Design review of the part built by this model. Coordinates are the model's own, in mm. Face numbers are marked on the shaded views. Coordinates: 2 decimals unless noted, no trailing zeros. Loops run counter-clockwise (first coordinate to the right, second up) from the corner with the lowest first, then second, coordinate; pieces in that order, holes last. Notation, with made-up numbers: (24, 15) -> (56, 15) arc R28 cw to (56, 34) -> close; hole circle Ø4 at (-32.75, 84). An arc over 180 degrees is marked (long way). One line per item, written item: value. Start each with the question number.
1. Insertion check: pin 1 (1.2 mm diameter, centred on x = 2.67, z = -5.07, fed in from +Y). The pin has a flat end and moves straight along its axis. Give the tip position at first contact, or say it passes through.
2. For probe 1 along Z at (x, y) = (2.6, 0.85); probe 2 along Z at (x, y) = (2.45, 1.7); probe 3 along X at (y, z) = (2.45, -25), list the stretches that pass through material, from the lowest coordinate up.
3. Add section C-C on y = 2.55. Write out the cut boundary in (x, z).
4. Add section B-B on x = 2.6. Write out the cut boundary in (y, z).
5. Draft analysis for pull direction Z (two halves, no side actions). For the marked faces 1, 2 and 3, state which applies: pulls with the +Z half, pulls with the -Z half, needs draft (parallel to the pull), parting line crosses it, or undercut.
6. Add section A-A on z = -25. Write out the cut boundary in (x, y).
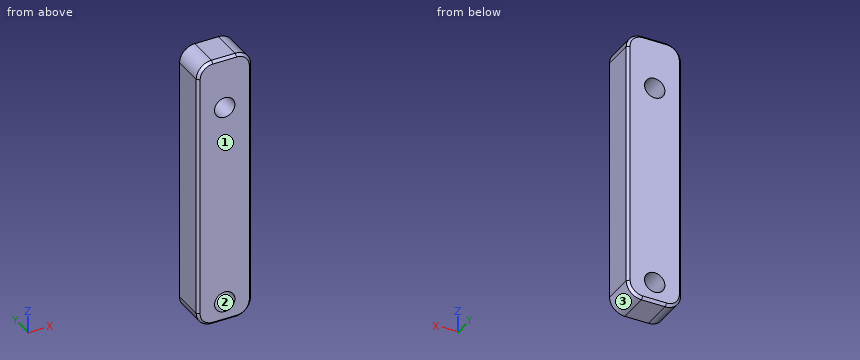
```python
from build123d import *

# Parameters (mm, degrees)
SKETCH_1_W          = 5.332575
SKETCH_1_H          = 27
EXTRUDE_1_DEPTH     = 3.5
FILLET_1_R          = 1.5
SKETCH_2_R          = 1
CUT_EXTRUDE_1_DEPTH = 4.5
CHAMFER_1_SIZE      = 0.25


with BuildPart() as part:
    # ｽｹｯﾁ1 → ﾎﾞｽ - 押し出し1 (new body)
    with BuildSketch(Plane(origin=(0, 0, 0), x_dir=(1, 0, 0), z_dir=(0, 1, 0))):
        with Locations((2.6662875, 13.5)):
            Rectangle(SKETCH_1_W, SKETCH_1_H)
    extrude(amount=EXTRUDE_1_DEPTH)

    # ﾌｨﾚｯﾄ1
    fillet_1_edges = [part.edges().sort_by_distance(p)[0] for p in [
        (5.332575, 1.75, -27),
        (5.332575, 1.75, 0),
        (0, 1.75, 0),
        (0, 1.75, -27),
    ]]
    fillet(fillet_1_edges, radius=FILLET_1_R)

    # ｽｹｯﾁ2 → ｶｯﾄ - 押し出し1 (cut, through all)
    with BuildSketch(Plane(origin=(0, 3.5, 0), x_dir=(1, 0, 0), z_dir=(0, 1, 0))):
        with Locations((2.6662875, 25)):
            Circle(SKETCH_2_R)
        with Locations((2.6662875, 5.06736)):
            Circle(SKETCH_2_R)
    extrude(amount=-CUT_EXTRUDE_1_DEPTH, mode=Mode.SUBTRACT)

    # 面取り1
    chamfer_1_edges = [part.edges().sort_by_distance(p)[0] for p in [
        (5.332575, 0, -13.5),
        (5.332575, 3.5, -13.5),
        (2.6662875, 0, -27),
        (2.6662875, 0, 0),
        (0, 0, -13.5),
        (4.893235172, 0, -26.560660172),
        (0.439339828, 0, -26.560660172),
        (0.439339828, 0, -0.439339828),
        (4.893235172, 0, -0.439339828),
        (2.6662875, 3.5, 0),
        (2.6662875, 3.5, -27),
        (0, 3.5, -13.5),
        (4.893235172, 3.5, -26.560660172),
        (0.439339828, 3.5, -26.560660172),
        (0.439339828, 3.5, -0.439339828),
        (4.893235172, 3.5, -0.439339828),
    ]]
    chamfer(chamfer_1_edges, length=CHAMFER_1_SIZE)


solid = part.part
```
Worked answers:
1. pin 1: passes through
2. probe 1: z = -27 to -26, -24 to -6.07, -4.07 to 0
2. probe 2: z = -27 to -25.98, -24.02 to -6.04, -4.09 to 0
2. probe 3: x = 0 to 1.67, 3.67 to 5.33
3. outline: (0, -25.5) arc R1.5 ccw to (1.5, -27) -> (3.83, -27) arc R1.5 ccw to (5.33, -25.5) -> (5.33, -1.5) arc R1.5 ccw to (3.83, 0) -> (1.5, 0) arc R1.5 ccw to (0, -1.5) -> close; hole circle Ø2 at (2.67, -25); hole circle Ø2 at (2.67, -5.07)
4. outline: (0, -26.75) -> (0.25, -27) -> (3.25, -27) -> (3.5, -26.75) -> (3.5, -26) -> (0, -26) -> close; (0, -24) -> (3.5, -24) -> (3.5, -6.07) -> (0, -6.07) -> close; (0, -4.07) -> (3.5, -4.07) -> (3.5, -0.25) -> (3.25, 0) -> (0.25, 0) -> (0, -0.25) -> close
5. face 1: needs draft
5. face 2: undercut
5. face 3: pulls with the -Z half
6. outline: (0, 0.25) -> (0.25, 0) -> (1.67, 0) -> (1.67, 3.5) -> (0.25, 3.5) -> (0, 3.25) -> close; (3.67, 0) -> (5.08, 0) -> (5.33, 0.25) -> (5.33, 3.25) -> (5.08, 3.5) -> (3.67, 3.5) -> close
